Can you work these out from the model? Positions are in its coordinate system, mm. A direction names the side the tool comes from. Give positions to 0.01 mm unless a question says otherwise; leave off trailing zeros. Loops run counter-clockwise (first coordinate to the right, second up) from the corner with the lowest first, then second, coordinate; pieces in that order, holes last.
from build123d import *

# Parameters (mm, degrees)
FILLET_1_R = 5
FILLET_2_R = 1


with BuildPart() as part:
    # 草圖1 → 旋轉1 (revolve)
    with BuildSketch(Plane.XY, mode=Mode.PRIVATE) as revolve_1_sk:
        Polygon((0, 0), (0, 40), (25, 40), (25, 20), (2, 20), (2, 2), (17, 0), align=None)
    revolve(revolve_1_sk.sketch.rotate(Axis((0, 0, 0), (0, 1, 0)), 90), axis=Axis((0, 0, 0), (0, 1, 0)))

    # 圓角1
    fillet_1_edges = [part.edges().sort_by_distance(p)[0] for p in [
        (0, 20, 25),
    ]]
    fillet(fillet_1_edges, radius=FILLET_1_R)

    # 圓角2
    fillet_2_edges = [part.edges().sort_by_distance(p)[0] for p in [
        (0, 2, 2),
    ]]
    fillet(fillet_2_edges, radius=FILLET_2_R)

    # 草圖2 → 除料-旋轉1 (revolve, cut)
    with BuildSketch(Plane.XY, mode=Mode.PRIVATE) as cut_revolve_1_sk:
        with BuildLine():
            Line((23, 40), (0, 40))
            Line((0, 40), (0, 22))
            Line((0, 22), (20, 22))
            ThreePointArc((20, 22), (22.121320344, 22.878679656), (23, 25))
            Line((23, 25), (23, 40))
        make_face()
    revolve(cut_revolve_1_sk.sketch.rotate(Axis((0, 40, 0), (0, -1, 0)), 90), axis=Axis((0, 40, 0), (0, -1, 0)), mode=Mode.SUBTRACT)


solid = part.part
(1) Suppose I cut it at A-A on y = 34. List the corners of the cut face in (x, z) for me.
Returned:
outline: circle Ø50 at (0, 0); hole circle Ø46 at (0, 0)
(2) Which directions (+Z, -Z, +X, -X, +Y, -Y) give clear straight access to the entire face, cutting with the end or side of a thin tool? Please do faces 4 (the cylindrical face through (2, 11, 0)), 5 (the flat face through (0, 22, 0)), 6 (the cylindrical face through (-7.509, 32.395, -23.846)).
Returned:
face 4: none
face 5: +Y
face 6: +Y, -Y
(3) Will these pins go through, and if not, where does the flat tip stop? P1, Ø4, axis at x = 5, y = 6.5, coming from the -Z side; P2, Ø4, axis at x = 16, y = 31.5, coming from the -Z side; P3, Ø5, axis at x = -14.5, z = -1, coming from the +Y side; P4, Ø8, axis at x = 2.5, z = -5.5, coming from the -Y side.
Returned:
P1: passes through
P2: stops at z = -20.71
P3: stops at y = 22
P4: stops at y = 0
(4) Please list where these lines run through material, in increasing order: probe 1 along X at (y, z) = (30, 0); probe 2 along Y at (x, z) = (-8.5, 17.5); probe 3 along Y at (x, z) = (-11.5, -1).
Returned:
probe 1: x = -25 to -23, 23 to 25
probe 2: y = 20 to 22
probe 3: y = 0 to 0.73, 20 to 22
(5) Thinking about a two-plate mould opening in Z: for faces 1 (the flat face through (7.3, 40, 22.1)), 2 (the cylindrical face through (-22.804, 32.605, -2.994)), 3 (the conical face through (3.663, 1.766, 0.813)), which applies, pulls with the +Z half, pulls with the -Z half, needs draft (parallel to the pull), parting line crosses it, or undercut?
Returned:
face 1: needs draft
face 2: undercut
face 3: parting line crosses it
(6) Suppose I cut it at B-B on y = 7. List the corners of the cut face in (x, z) for me.
Returned:
outline: circle Ø4 at (0, 0)
